Input: part model. Units: mm. Frame: model coordinates. Face numbers are marked on the shaded views. A direction names the side the tool comes from. Round coordinates to 2 decimals unless told otherwise and drop trailing zeros. Loops run counter-clockwise (first coordinate to the right, second up) from the corner with the lowest first, then second, coordinate; pieces in that order, holes last. Notation, with made-up numbers: (-24.75, -3) - (18.25, -3) arc R27 cw to (18.25, 26) - close; hole circle Ø7 at (-29.5, 74.25). An arc over 180 degrees is marked (long way). Write each question's results on one line, items separated by ' | '.
Autodesk Inventor part; units mm, degrees
ref_plane "YZ Plane" through (0, 0, 0) normal (1, 0, 0) x (0, 1, 0)
ref_plane "XZ Plane" through (0, 0, 0) normal (0, 1, 0) x (-1, 0, 0)
ref_plane "XY Plane" through (0, 0, 0) normal (0, 0, 1) x (1, 0, 0)
sketch "Sketch1" plane through (0, 0, 0) normal (0, 1, 0) x (-1, 0, 0)
  circle A0 centre (0, 0) radius 14.5
  dimension "d0" = 29
extrude "Extrusion1" add sketch "Sketch1" along normal blind 14
sketch "Sketch2" plane through (0, 0, 0) normal (1, 0, 0) x (0, 1, 0)
  line L0 (14, -14.5) -> (14, 14.5)
  line L1 (14, 0) -> (14, -25)
  line L2 (14, -25) -> (7.1034, -25)
  line L3 (7.1034, -25) -> (14, 0)
  line L4 (5, -14.5) -> (5, -13.5)
  line L5 (5, -13.5) -> (8, -13.5)
  line L6 (8, -13.5) -> (8, -14.5)
  line L7 (8, -14.5) -> (5, -14.5)
  line L8 (1, -13.5) -> (3, -13.5)
  line L9 (3, -13.5) -> (3, -14.5)
  line L10 (3, -14.5) -> (1, -14.5)
  line L11 (1, -14.5) -> (1, -13.5)
  line L12 (0, 14.5) -> (0, -14.5)
  line L13 (0, -14.5) -> (14, -14.5)
  line L14 (-2.8, 0) -> (16.8, 0)
  point P0 (0, 0)
  point P1 (10, -14.5)
  dimension "d3" = 1
  dimension "d4" = 3
  dimension "d5" = 2
  dimension "d6" = 1
  dimension "d7" = 2
  dimension "d8" = 1
  dimension "d9" = 2
  dimension "d10" = 25
revolve "Revolution1" cut sketch "Sketch2" angle 360 about axis through (0, -10, 0) along (0, 1, 0) contours L13 L3 L0 | L1 L2 L3 L13 | L7 L4 L5 L6 | L11 L8 L9 L10
sketch "Sketch3" plane through (0, 0, 0) normal (1, 0, 0) x (0, 1, 0)
  line L0 (0, 0) -> (0, 8)
  line L1 (0, 8) -> (4, 8)
  line L2 (4, 8) -> (4, 13.7374)
  line L3 (4, 13.7374) -> (9, 0)
  line L4 (9, 0) -> (0, 0)
  line L5 (9, 0) -> (9, 10.144) construction
  line L6 (0, 14.5) -> (0, -14.5) construction
  line L7 (-2.8, 0) -> (16.8, 0) construction
  point P0 (0, 0)
  dimension "d12" = 8
  dimension "d13" = 4
  dimension "d14" = 5
  dimension "d15" = 20
  dimension "d19" = 10.144
revolve "Revolution2" cut sketch "Sketch3" angle 360 about axis through (0, -10, 0) along (0, 1, 0)
properties part number "Valvula"
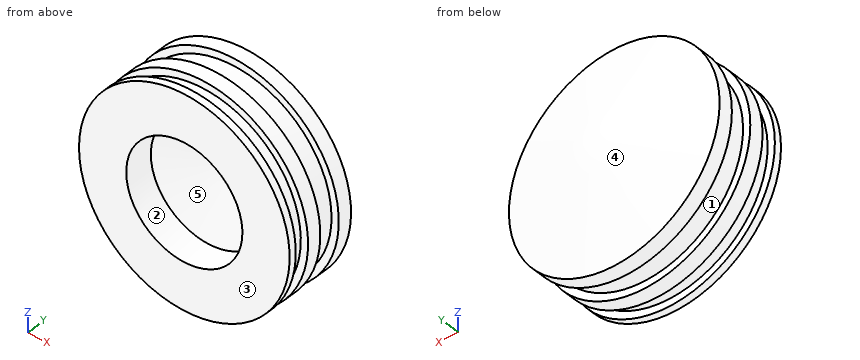
1. Section query C-C, the plane y = 6. Output: boundary loops of the cut face in (x, z), plus the area to 3 significant figures.
Answer:
outline: circle Ø27 at (0, 0); hole circle Ø16.48 at (0, 0) | area: 359 mm^2
2. Contact query for flat-ended pins moving along their axis: pin 1 (3 mm diameter, centred on x = 9.5, z = 4.5, fed in from +Y); pin 2 (8 mm diameter, centred on x = -3.5, z = 6, fed in from +Y); pin 3 (8.5 mm diameter, centred on x = 0.5, z = -1, fed in from -Y). Output: stop coordinate, or through.
Answer:
pin 1: y = 11.51 | pin 2: y = 13.19 | pin 3: y = 7.05
3. Section query A-A, the plane y = 2. Output: boundary loops of the cut face in (x, z).
Answer:
outline: circle Ø27 at (0, 0); hole circle Ø16 at (0, 0)
4. Section query B-B, the plane y = 12.5. Output: boundary loops of the cut face in (x, z), plus the area to 3 significant figures.
Answer:
outline: circle Ø10.87 at (0, 0) | area: 92.9 mm^2
5. Mould query, pull axis Z, two halves, no side actions, for the marked faces 3, 4 and 5. Classes: pulls with the +Z half, pulls with the -Z half, needs draft (parallel to the pull), parting line crosses it, or undercut.
Answer:
face 3: needs draft | face 4: parting line crosses it | face 5: undercut
6. Line query: line 1 (X direction, y = 3.05, z = 0); line 2 (X direction, y = 1.7, z = 0); line 3 (Z direction, x = -1.75, y = 2.5). Output: solid intervals per line, ascending. Write a range as [from, to].
Answer:
line 1: [-14.5, -8], [8, 14.5] | line 2: [-13.5, -8], [8, 13.5] | line 3: [-13.39, -7.81], [7.81, 13.39]
7. Set-up query: the marked faces 1 and 2. Return all of +Z, -Z, +X, -X, +Y, -Y with unobstructed straight access to the full face (end or side cutting, diameter ignored); none if empty.
Answer:
face 1: none | face 2: -Y
